Verification items for this drawing (mm, ordinates from the low corner). A direction names the side the tool comes from. Coordinates: 2 decimals unless noted, no trailing zeros. Loops run counter-clockwise (first coordinate to the right, second up) from the corner with the lowest first, then second, coordinate; pieces in that order, holes last. Notation, with made-up numbers: (29, 32) -> (82, 32) arc R29 ccw to (82, 69) -> close; hole circle Ø4 at (50, 46.25). An arc over 180 degrees is marked (long way). Write item = value, one per line.
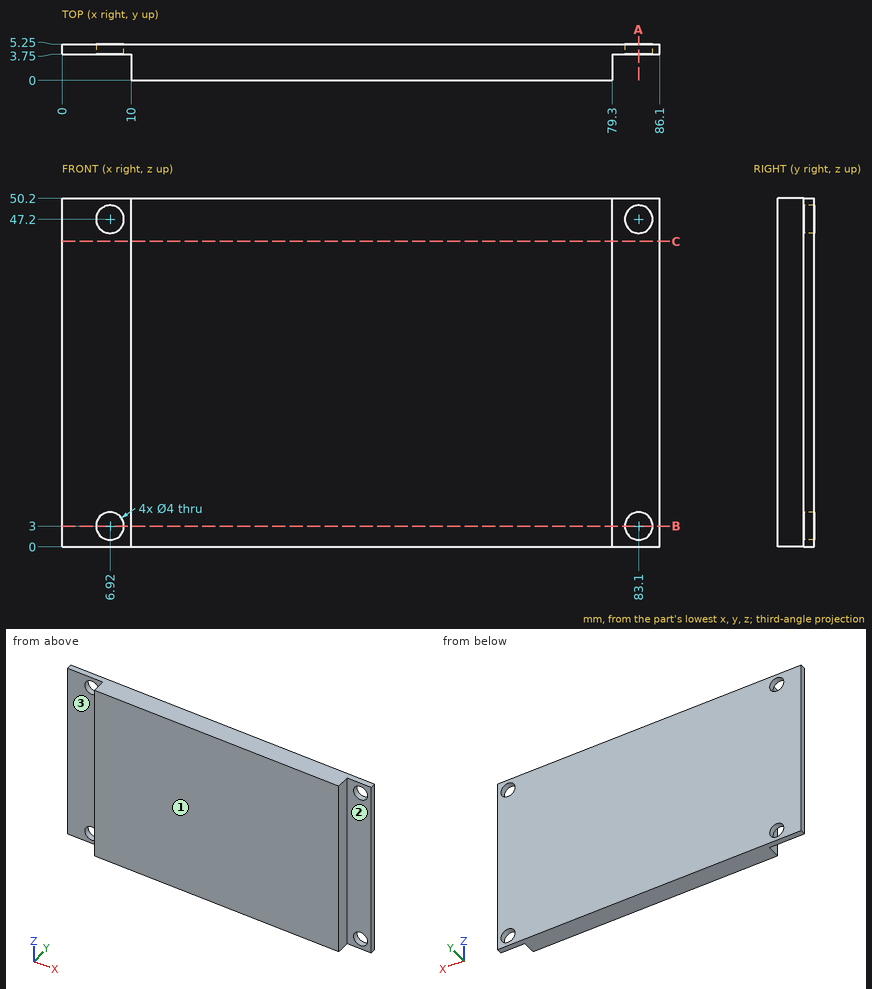
1) Depth check by flat-ended pin: pin 1 Ø1.9 at (y, z) = (2, 36.5) entering from -X; pin 2 Ø2 at (x, z) = (81.5, 26) entering from -Y; pin 3 Ø2.5 at (x, z) = (83.1, 3) entering from +Y; pin 4 Ø1.9 at (y, z) = (2, 16.5) entering from +X. Enter the tip coordinate at first touch or a pass-through.
Ans:
pin_1 = 10
pin_2 = 3.75
pin_3 = through
pin_4 = 79.3
2) Sectioned sample at C-C, the plane z = 44. Record the cut outline in (x, y).
Ans:
outline = (0, 3.75) -> (10, 3.75) -> (10, 0) -> (79.3, 0) -> (79.3, 3.75) -> (86.1, 3.75) -> (86.1, 5.25) -> (0, 5.25) -> close
3) Sectioned sample at B-B, the plane z = 3. Record the cut outline in (x, y).
Ans:
outline = (0, 3.75) -> (4.92, 3.75) -> (4.92, 5.25) -> (0, 5.25) -> close; (8.92, 3.75) -> (10, 3.75) -> (10, 0) -> (79.3, 0) -> (79.3, 3.75) -> (81.1, 3.75) -> (81.1, 5.25) -> (8.92, 5.25) -> close; (85.1, 3.75) -> (86.1, 3.75) -> (86.1, 5.25) -> (85.1, 5.25) -> close
4) Material ranges on line 1 (Z direction, x = 83.1, y = 4.8); line 2 (Y direction, x = 5, z = 33.5); line 3 (X direction, y = 2.2, z = 42.5), recorded low to high.
Ans:
line_1 = 0 to 1, 5 to 45.2, 49.2 to 50.2
line_2 = 3.75 to 5.25
line_3 = 10 to 79.3
5) Tool access check on the marked faces 1, 2 and 3. Record the directions out of +Z, -Z, +X, -X, +Y, -Y that give a thin tool (end or side, any length) a straight path to the whole face; none if there is none.
Ans:
face_1 = +Z, -Z, +X, -X, -Y
face_2 = +Z, -Z, +X, -Y
face_3 = +Z, -Z, -X, -Y
6) Sectioned sample at A-A, the plane x = 83.1. Record the cut outline in (y, z).
Ans:
outline = (3.75, 0) -> (5.25, 0) -> (5.25, 1) -> (3.75, 1) -> close; (3.75, 5) -> (5.25, 5) -> (5.25, 45.2) -> (3.75, 45.2) -> close; (3.75, 49.2) -> (5.25, 49.2) -> (5.25, 50.2) -> (3.75, 50.2) -> close
